Source: CAD feature listing. Evaluate the final solid. Frame: model axes, mm. A direction names the side the tool comes from. Give positions to 0.01 mm unless a question says otherwise; leave off trailing zeros. Order: outer loops, then holes, each group sorted by start corner. A loop starts at its lowest first (then second) coordinate and runs counter-clockwise, first axis right, second up. Notation, with made-up numbers: M 81.25,65.25 L 92.25,65.25 A24 cw 92.25,79.25 Z; hole C -34.5,18.25 d11. An arc over 180 degrees is marked long. Use CSV: the item, a comma, the result in double quotes. Start each with the question number.
Item 1: Ray query, probe 1 along X at (y, z) = (-18.55, 4.4); probe 2 along X at (y, z) = (-20.9, -1.5); probe 3 along Y at (x, z) = (-8.5, 1). Return the intervals inside material, ascending. Write a range as from..to.
Item 2: Access query for faces 1 (the face through (2, -18.7, -4)), 2 (the face through (5.67, -21.62, 1.77)), 3 (the face through (-7, -18, -5)). Directions: +Z, -Z, +X, -X, +Y, -Y. A direction counts if a zero-diameter tool reaches every point of the face in a straight line with its end or side. Return the directions, or none.
Item 3: Section query C-C on z = -4.5. Return loops of the section in (x, y), and give its area (3 significant figures).
Item 4: Section query A-A on x = -0.4. Return loops of the section in (y, z), and give its area (3 significant figures).
Item 5: First-contact query: pin 1 (0.7 mm diameter, centred on y = -19, z = -3.5, fed in from +X); pin 2 (3.5 mm diameter, centred on x = -7.5, z = 5, fed in from +Y); pin 3 (1.2 mm diameter, centred on x = 7, y = -21, fed in from +Z). Flat tips, straight axial feed; report the tip coordinate or a pass-through.
Item 6: Section query B-B on x = -7.6. Return loops of the section in (y, z), and give its area (3 significant figures).
from build123d import *

# Parameters (mm, degrees)
SKETCH_1_R          = 2.4
EXTRUDE_1_DEPTH     = 11.5
SKETCH_1_7_W        = 0.5
SKETCH_1_7_H        = 1.8
EXTRUDE_3_DEPTH     = 1.1
EXTRUDE_START       = -13.8
SKETCH_1_8_W        = 0.5
SKETCH_1_8_H        = 1.8
EXTRUDE_4_DEPTH     = 14.9
EXTRUDE_5_DEPTH     = 1.3
SKETCH_3_W          = 0.6
SKETCH_3_H          = 0.6
EXTRUDE_6_DEPTH     = 3.9
SKETCH_3_3_W        = 0.6
SKETCH_3_3_H        = 3
EXTRUDE_7_DEPTH     = 3
EXTRUDE_START_2     = -3
SKETCH_4_W          = 6.9
SKETCH_4_H          = 3.9
EXTRUDE_8_DEPTH     = 0.3
SKETCH_6_W          = 12.5
SKETCH_6_H          = 7.5
CUT_EXTRUDE_1_DEPTH = 0.7
EXTRUDE_START_3     = -1.3
SKETCH_5_R          = 0.7
EXTRUDE_9_DEPTH     = 0.4
SKETCH_7_R          = 0.9
SKETCH_7_R_2        = 0.8
EXTRUDE_10_DEPTH    = 12.5
SKETCH_8_R          = 0.5
EXTRUDE_11_DEPTH    = 0.6
SKETCH_9_W          = 55.778584291
SKETCH_9_H          = 36.536448335
CUT_EXTRUDE_2_DEPTH = 23.165964901


with BuildPart() as part:
    # 草图1 → 凸台-拉伸1 (new body)
    with BuildSketch(Plane(origin=(0, 0, 0), x_dir=(0, 0, -1), z_dir=(1, 0, 0))):
        Circle(SKETCH_1_R)
    extrude(amount=EXTRUDE_1_DEPTH)

    # 草图1<7> → 凸台-拉伸3 (add)
    with BuildSketch(Plane(origin=(0, 0, 0), x_dir=(0, 0, -1), z_dir=(1, 0, 0))):
        with BuildLine():
            Line((5, -0.6), (2.323790008, -0.6))
            ThreePointArc((2.323790008, -0.6), (1.469693849, -1.897366594), (8e-09, -2.4))
            Line((8e-09, -2.4), (5, -2.4))
            Line((5, -2.4), (5, -0.6))
        make_face()
        with BuildLine():
            Line((-2.323790008, -0.6), (-2.4, -0.6))
            Line((-2.4, -0.6), (-2.4, -2.4))
            Line((-2.4, -2.4), (8e-09, -2.4))
            ThreePointArc((8e-09, -2.4), (-1.469693842, -1.897366599), (-2.323790008, -0.6))
        make_face()
        with Locations((-2.65, -1.5)):
            Rectangle(SKETCH_1_7_W, SKETCH_1_7_H)
        with BuildLine():
            Line((5, 2), (1.326649916, 2))
            ThreePointArc((1.326649916, 2), (2.114705629, 1.134909732), (2.4, 0))
            ThreePointArc((2.4, 0), (2.380871271, -0.302410302), (2.323790008, -0.6))
            Line((2.323790008, -0.6), (5, -0.6))
            Line((5, -0.6), (5, 2))
        make_face()
        with BuildLine():
            ThreePointArc((-2.323790008, -0.6), (-2.380871271, -0.302410299), (-2.4, 5e-09))
            Line((-2.4, 5e-09), (-2.4, -0.6))
            Line((-2.4, -0.6), (-2.323790008, -0.6))
        make_face()
    extrude(amount=EXTRUDE_3_DEPTH)

    # 草图1<8> → 凸台-拉伸4 (add)
    with BuildSketch(Plane(origin=(0, 0, 0), x_dir=(0, 0, -1), z_dir=(1, 0, 0)).offset(EXTRUDE_START)):
        with BuildLine():
            Line((5, -0.6), (2.323790008, -0.6))
            ThreePointArc((2.323790008, -0.6), (1.469693849, -1.897366594), (8e-09, -2.4))
            Line((8e-09, -2.4), (5, -2.4))
            Line((5, -2.4), (5, -0.6))
        make_face()
        with BuildLine():
            Line((2.323790008, -0.6), (-2.323790008, -0.6))
            ThreePointArc((-2.323790008, -0.6), (-1.469693842, -1.897366599), (8e-09, -2.4))
            ThreePointArc((8e-09, -2.4), (1.469693849, -1.897366594), (2.323790008, -0.6))
        make_face()
        with BuildLine():
            Line((-2.323790008, -0.6), (-2.4, -0.6))
            Line((-2.4, -0.6), (-2.4, -2.4))
            Line((-2.4, -2.4), (8e-09, -2.4))
            ThreePointArc((8e-09, -2.4), (-1.469693842, -1.897366599), (-2.323790008, -0.6))
        make_face()
        with Locations((-2.65, -1.5)):
            Rectangle(SKETCH_1_8_W, SKETCH_1_8_H)
    extrude(amount=EXTRUDE_4_DEPTH)

    # 草图1<9> → 凸台-拉伸5 (add)
    with BuildSketch(Plane(origin=(0, 0, 0), x_dir=(0, 0, -1), z_dir=(1, 0, 0)).offset(EXTRUDE_START)):
        with BuildLine():
            Line((5, 2), (1.326649916, 2))
            ThreePointArc((1.326649916, 2), (2.114705629, 1.134909732), (2.4, 0))
            ThreePointArc((2.4, 0), (2.380871271, -0.302410302), (2.323790008, -0.6))
            Line((2.323790008, -0.6), (5, -0.6))
            Line((5, -0.6), (5, 2))
        make_face()
        with BuildLine():
            Line((1.326649916, 2), (-1.326649916, 2))
            ThreePointArc((-1.326649916, 2), (-2.114705628, 1.134909735), (-2.4, 5e-09))
            ThreePointArc((-2.4, 5e-09), (-2.380871271, -0.302410299), (-2.323790008, -0.6))
            Line((-2.323790008, -0.6), (2.323790008, -0.6))
            ThreePointArc((2.323790008, -0.6), (2.380871271, -0.302410302), (2.4, 0))
            ThreePointArc((2.4, 0), (2.114705629, 1.134909732), (1.326649916, 2))
        make_face()
        with BuildLine():
            ThreePointArc((-2.323790008, -0.6), (-2.380871271, -0.302410299), (-2.4, 5e-09))
            Line((-2.4, 5e-09), (-2.4, -0.6))
            Line((-2.4, -0.6), (-2.323790008, -0.6))
        make_face()
    extrude(amount=EXTRUDE_5_DEPTH)

    # 草图3 → 凸台-拉伸6 (add)
    with BuildSketch(Plane.XY):
        with Locations((11.2, 0.8)):
            Rectangle(SKETCH_3_W, SKETCH_3_H)
        with Locations((11.2, -0.8)):
            Rectangle(SKETCH_3_W, SKETCH_3_H)
        with Locations((7.6, 0.8)):
            Rectangle(SKETCH_3_W, SKETCH_3_H)
        with Locations((7.6, -0.8)):
            Rectangle(SKETCH_3_W, SKETCH_3_H)
    extrude(amount=-EXTRUDE_6_DEPTH)

    # 草图3<3> → 凸台-拉伸7 (add)
    with BuildSketch(Plane.XY):
        with Locations((11.2, 0)):
            Rectangle(SKETCH_3_3_W, SKETCH_3_3_H)
        with Locations((7.6, 0)):
            Rectangle(SKETCH_3_3_W, SKETCH_3_3_H)
    extrude(amount=-EXTRUDE_7_DEPTH)

    # 草图4 → 凸台-拉伸8 (add)
    with BuildSketch(Plane.XY.offset(EXTRUDE_START_2)):
        with Locations((8.45, 0)):
            Rectangle(SKETCH_4_W, SKETCH_4_H)
    extrude(amount=EXTRUDE_8_DEPTH)

    # 草图6 → 切除-拉伸1 (cut)
    with BuildSketch(Plane(origin=(0, -0.6, 0), x_dir=(1, 0, 0), z_dir=(0, 1, 0))):
        with Locations((-6.25, 1.25)):
            Rectangle(SKETCH_6_W, SKETCH_6_H)
    extrude(amount=-CUT_EXTRUDE_1_DEPTH, mode=Mode.SUBTRACT)

    # 草图5 → 凸台-拉伸9 (add)
    # profile 1 of 3: a face of its own
    with BuildSketch(Plane(origin=(0, 0, 0), x_dir=(1, 0, 0), z_dir=(0, 1, 0)).offset(EXTRUDE_START_3)):
        with BuildLine():
            ThreePointArc((3.1, 2.8), (4.384523258, 5.074596669), (1.773350084, 5))
            Line((1.773350084, 5), (1.1, 5))
            Line((1.1, 5), (1.1, 2.8))
            Line((1.1, 2.8), (3.1, 2.8))
        make_face()
        with Locations(Location((3.1, 4.3, 0), (0, 0, 270))):
            Circle(SKETCH_5_R, mode=Mode.SUBTRACT)
    # profile 2 of 3: a face of its own
    with BuildSketch(Plane(origin=(0, 0, 0), x_dir=(1, 0, 0), z_dir=(0, 1, 0)).offset(EXTRUDE_START_3)):
        with BuildLine():
            Line((-6.1, -4.4), (-6.1, -2.9))
            Line((-6.1, -2.9), (-9.1, -2.9))
            Line((-9.1, -2.9), (-9.1, -4.4))
            ThreePointArc((-9.1, -4.4), (-7.6, -5.9), (-6.1, -4.4))
        make_face()
        with Locations(Location((-7.6, -4.4, 0), (0, 0, 270))):
            Circle(SKETCH_5_R, mode=Mode.SUBTRACT)
    # profile 3 of 3: a face of its own
    with BuildSketch(Plane(origin=(0, 0, 0), x_dir=(1, 0, 0), z_dir=(0, 1, 0)).offset(EXTRUDE_START_3)):
        with BuildLine():
            Line((-13.8, 5), (-15.6, 5))
            ThreePointArc((-15.6, 5), (-17.4, 3.2), (-15.6, 1.4))
            Line((-15.6, 1.4), (-13.8, 1.4))
            Line((-13.8, 1.4), (-13.8, 5))
        make_face()
        with Locations(Location((-15.6, 3.2, 0), (0, 0, 270))):
            Circle(SKETCH_5_R, mode=Mode.SUBTRACT)
    extrude(amount=-EXTRUDE_9_DEPTH)

    # 草图7 → 凸台-拉伸10 (add)
    with BuildSketch(Plane.ZY):
        with Locations(Location((0, 0, 0), (0, 0, 180))):
            Circle(SKETCH_7_R)
        with Locations(Location((-3.3, 0, 0), (0, 0, 180))):
            Circle(SKETCH_7_R_2)
    extrude(amount=EXTRUDE_10_DEPTH)

    # 草图8 → 凸台-拉伸11 (add)
    with BuildSketch(Plane.XZ.offset(2.4)):
        with Locations(Location((-12.3, -1.05, 0), (0, 0, 90))):
            Circle(SKETCH_8_R)
        with Locations(Location((-0.4, -1.05, 0), (0, 0, 90))):
            Circle(SKETCH_8_R)
    extrude(amount=EXTRUDE_11_DEPTH)


with BuildPart() as body_2:
    # 镜向2: mirrored copy
    add(part.part.mirror(Plane.ZX.offset(-10)))


with BuildPart() as part_1:
    add(part.part)

    # 草图9 → 切除-拉伸2 (cut, through all)
    with BuildSketch(Plane(origin=(0, -10, 0), x_dir=(1, 0, 0), z_dir=(0, 1, 0))):
        with Locations((1.175159636, 0.404925991)):
            Rectangle(SKETCH_9_W, SKETCH_9_H)
    extrude(amount=CUT_EXTRUDE_2_DEPTH, mode=Mode.SUBTRACT)


solid = body_2.part
Verdict:
1,probe 1,"-9.1..-8.3, -6.9..-6.1"
1,probe 2,"-13.8..-12.5, 0..11.5"
1,probe 3,"-18.7..-17.6"
2,face 1,"-Z, -Y"
2,face 2,"none"
2,face 3,"-Z, -X, +Y, -Y"
3,outline,"M -16.84,-18.7 L -13.8,-18.7 L -13.8,-22 L -12.5,-22 L -12.5,-18.7 L 0,-18.7 L 0,-22 L 1.1,-22 L 1.1,-18.7 L 2.43,-18.7 L 2.43,-18.3 L 1.1,-18.3 L 1.1,-17.6 L -13.8,-17.6 L -13.8,-18.3 L -16.84,-18.3 Z; M 3.77,-18.7 L 4.59,-18.7 L 4.59,-18.3 L 3.77,-18.3 Z"
3,area,"26.4 mm2"
4,outline,"C -20,0 d1.8; C -20,-3.3 d1.6; M -19.4,2.5 L -18.7,2.5 L -18.7,-5 L -17.6,-5 L -17.6,-1.55 L -17,-1.55 L -17,-0.55 L -17.6,-0.55 L -17.6,2.9 L -19.4,2.9 Z"
4,area,"14.1 mm2"
5,pin 1,"x = 11.5"
5,pin 2,"y = -18.3"
5,pin 3,"z = 2.37"
6,outline,"C -20,0 d1.8; C -20,-3.3 d1.6; M -19.4,2.5 L -18.7,2.5 L -18.7,-5 L -17.6,-5 L -17.6,2.9 L -18.3,2.9 L -18.3,3.7 L -18.7,3.7 L -18.7,2.9 L -19.4,2.9 Z; M -18.7,5.1 L -18.3,5.1 L -18.3,5.9 L -18.7,5.9 Z"
6,area,"14.2 mm2"
